from build123d import *

# Parameters (mm, degrees)
SKETCH2_W                      = 390
SKETCH2_H                      = 290
BOSS_EXTRUDE1_DEPTH            = 50
SHELL1_T                       = -20
SKETCH3_R                      = 20
BOSS_EXTRUDE2_DEPTH            = 50
F_15_0_15_DIAMETER_HOLE1_D     = 15
F_15_0_15_DIAMETER_HOLE1_DEPTH = 20
F_15_0_15_DIAMETER_HOLE1_TIP   = 4.506454643


with BuildPart() as part:
    # Sketch2 → Boss-Extrude1 (new body)
    with BuildSketch(Plane(origin=(0, 0, 0), x_dir=(1, 0, 0), z_dir=(0, 1, 0))):
        Rectangle(SKETCH2_W, SKETCH2_H)
    extrude(amount=BOSS_EXTRUDE1_DEPTH)

    # Shell1
    shell1_openings = [part.faces().sort_by_distance(p)[0] for p in [
        (0, 50, 0),
    ]]
    offset(amount=SHELL1_T, openings=shell1_openings, kind=Kind.INTERSECTION)

    # Sketch3 → Boss-Extrude2 (add)
    with BuildSketch(Plane(origin=(0, 50, 0), x_dir=(1, 0, 0), z_dir=(0, 1, 0))):
        with Locations((-195, 145)):
            Circle(SKETCH3_R)
        with Locations((195, 145)):
            Circle(SKETCH3_R)
        with Locations((195, -145)):
            Circle(SKETCH3_R)
        with Locations((-195, -145)):
            Circle(SKETCH3_R)
    extrude(amount=-BOSS_EXTRUDE2_DEPTH)

    # Ø15.0 (15) Diameter Hole1
    with Locations(Plane(origin=(0, 50, 0), x_dir=(1, 0, 0), z_dir=(0, 1, 0))):
        with Locations((-195, 145), (195, 145), (195, -145), (-195, -145)):
            Hole(F_15_0_15_DIAMETER_HOLE1_D / 2, depth=F_15_0_15_DIAMETER_HOLE1_DEPTH)
            with Locations((0, 0, -(F_15_0_15_DIAMETER_HOLE1_DEPTH + F_15_0_15_DIAMETER_HOLE1_TIP / 2))):  # 118° drill point
                Cone(0, F_15_0_15_DIAMETER_HOLE1_D / 2, F_15_0_15_DIAMETER_HOLE1_TIP, mode=Mode.SUBTRACT)


solid = part.part
The listing builds one solid part. Answer for the finished solid, in the listing's coordinates (mm). A direction names the side the tool comes from. Coordinates: 2 decimals unless noted, no trailing zeros. Loops run counter-clockwise (first coordinate to the right, second up) from the corner with the lowest first, then second, coordinate; pieces in that order, holes last. Notation, with made-up numbers: (10.5, 59.5) -> (18.5, 59.5) arc R17 cw to (18.5, 72.5) -> close; hole circle Ø3 at (33, -8). An arc over 180 degrees is marked (long way). Write item = value, one per line. Start each with the question number.
1) Straight lines are drawn through the part: line 1 (X direction, y = 21.5, z = -115.5); line 2 (Z direction, x = -93.5, y = 28.5); line 3 (Y direction, x = 65, z = -12). For each, find the intervals that lie inside material, in ascending order. Write a range as from..to.
2) A tool of negligible diameter and unlimited length cuts with its end or side. For faces 1 (the face through (-2, 25, -145)), 2 (the face through (-208.67, 25.35, -159.6)), 3 (the face through (-2, 25, 145)), 4 (the face through (-195, 25, 2)), 5 (the face through (-202.154, 39.86, -147.253)), from which of +Z, -Z, +X, -X, +Y, -Y can it reach the whole face along a straight path? Write none if from no direction.
3) A cutting plane is placed at C-C (x = 110). Give the vertices of the cut face in (y, z), then the cut area to 3 significant figures.
4) The mould has two halves that part along X. Classify faces 6 (the face through (195, 25, 2)), 7 (the face through (175, 35, 2)), 8 (the face through (-33, 50, -135)): released by +X, released by -X, zero draft, split by the parting line, or undercut.
5) Given pin 1 Ø10 at (y, z) = (42.5, 116) entering from -X; pin 2 Ø15 at (y, z) = (35, -33) entering from +X; pin 3 Ø25 at (x, y) = (8.5, 25) entering from +Z, each flat-ended and moving along its own axis, determine where each tip first touches the part or whether it passes through.
6) A cutting plane is placed at A-A (y = 37.5). Give the vertices of the cut face in (x, z).
7) A cutting plane is placed at B-B (z = 58.5). Give the vertices of the cut face in (x, y).
Responses:
q1.line_1 = -195..-175, 175..195
q1.line_2 = -145..-125, 125..145
q1.line_3 = 0..20
q2.face_1 = -Z, +Y, -Y
q2.face_2 = +Y, -Y
q2.face_3 = +Z, +Y, -Y
q2.face_4 = -X, +Y, -Y
q2.face_5 = +Y
q3.outline = (0, -145) -> (50, -145) -> (50, -125) -> (20, -125) -> (20, 125) -> (50, 125) -> (50, 145) -> (0, 145) -> close
q3.area = 7,000 mm²
q4.face_6 = released by +X
q4.face_7 = undercut
q4.face_8 = zero draft
q5.pin_1 = -195
q5.pin_2 = 195
q5.pin_3 = 145
q6.outline = (-195, -125) arc R20 ccw (long way) to (-175, -145) -> (175, -145) arc R20 ccw (long way) to (195, -125) -> (195, 125) arc R20 ccw (long way) to (175, 145) -> (-175, 145) arc R20 ccw (long way) to (-195, 125) -> close; hole circle Ø15 at (-195, -145); hole circle Ø15 at (-195, 145); hole (-175, -125) -> (175, -125) -> (175, 125) -> (-175, 125) -> close; hole circle Ø15 at (195, -145); hole circle Ø15 at (195, 145)
q7.outline = (-195, 0) -> (195, 0) -> (195, 50) -> (175, 50) -> (175, 20) -> (-175, 20) -> (-175, 50) -> (-195, 50) -> close
